from build123d import *

# Parameters (mm, degrees)
F0_R     = 2
F1_DEPTH = 10
F4_SIZE  = 0.5
F6_DEPTH = 0.56


with BuildPart() as f1:
    # F0 (on Top) → F1 (new body)
    with BuildSketch(Plane.XY):
        Circle(F0_R)
    extrude(amount=F1_DEPTH)

    # F2 (on Right) → F3 (revolve, cut)
    with BuildSketch(Plane.YZ):
        Polygon((0, 10.2037759498), (-2.4595215172, 10.2037759498), (-2.4595215172, 7.5622705054), (0, 10.0217920226), align=None)
    revolve(axis=Axis((0, 0, 10.1127839862), (0, 0, -1)), mode=Mode.SUBTRACT)

    # F4
    f4_edges = [f1.edges().sort_by_distance(p)[0] for p in [
        (-2, 0, 0),
    ]]
    chamfer(f4_edges, length=F4_SIZE)

    # F5 (on face) → F6 (cut)
    with BuildSketch(Plane(origin=(0, 0, 0), x_dir=(1, 0, 0), z_dir=(0, 0, -1))):
        with BuildLine():
            ThreePointArc((-0.125, 1.4947825929), (0, 1.5), (0.125, 1.4947825929))
            Line((0.125, 1.4947825929), (0.125, 2.363476136))
            Line((0.125, 2.363476136), (-0.125, 2.363476136))
            Line((-0.125, 2.363476136), (-0.125, 1.4947825929))
        make_face()
        with BuildLine():
            ThreePointArc((-0.125, -1.4947825929), (0, -1.5), (0.125, -1.4947825929))
            Line((0.125, -1.4947825929), (0.125, 1.4947825929))
            ThreePointArc((0.125, 1.4947825929), (0, 1.5), (-0.125, 1.4947825929))
            Line((-0.125, 1.4947825929), (-0.125, -1.4947825929))
        make_face()
        with BuildLine():
            Line((-0.125, -2.363476136), (0.125, -2.363476136))
            Line((0.125, -2.363476136), (0.125, -1.4947825929))
            ThreePointArc((0.125, -1.4947825929), (0, -1.5), (-0.125, -1.4947825929))
            Line((-0.125, -1.4947825929), (-0.125, -2.363476136))
        make_face()
    extrude(amount=-F6_DEPTH, mode=Mode.SUBTRACT)


solid = f1.part
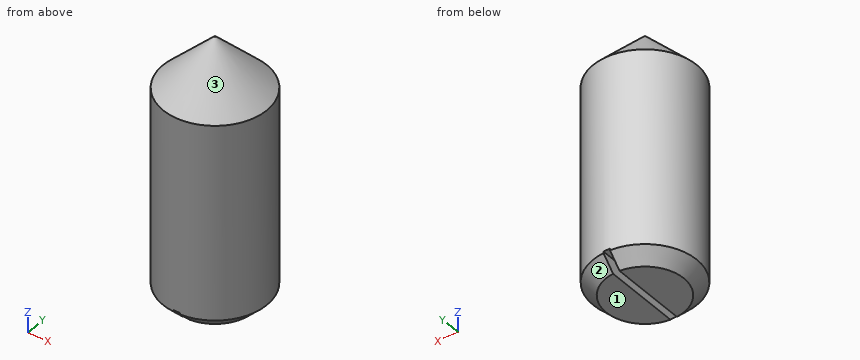
Build history of the part. All positions in model axes, mm. Face numbers are marked on the shaded views. Give positions to 0.01 mm unless a question says otherwise; leave off trailing zeros. Order: outer loops, then holes, each group sorted by start corner. A loop starts at its lowest first (then second) coordinate and runs counter-clockwise, first axis right, second up. Notation, with made-up numbers: M 61.25,33.5 L 98.25,33.5 A8 cw 98.25,43.5 Z; hole C -7,51 d10. An arc over 180 degrees is marked long. Put each result on its own line as item: value.
Item 1: Cut at A-A on z = 3. Write the cut outline in (x, y).
Results are:
outline: C 0,0 d4
Item 2: Drop a flat-ended pin along its axis: pin 1 Ø1 at (x, y) = (1, 1) entering from +Z. Give the stop position or say it passes through.
Results are:
pin 1: z = 9.11
Item 3: Pull direction X, two halves, no side cores. Call the marked faces 1, 2 and 3: +X half, -X half, draft (parallel to the pull), parting line (faces both ways), or undercut.
Results are:
face 1: draft
face 2: +X half
face 3: parting line
Item 4: Wall check: probe 1 along X at (y, z) = (0.15, 5.25); probe 2 along X at (y, z) = (1.55, 6.5). Give the ranges that are in metal, low to high.
Results are:
probe 1: -1.99 to 1.99
probe 2: -1.26 to 1.26
